from build123d import *

# Parameters (mm, degrees)
SKETCH1_W           = 30
SKETCH1_H           = 15
BOSS_EXTRUDE1_DEPTH = 15
SKETCH2_W           = 28
SKETCH2_H           = 13
CUT_EXTRUDE1_DEPTH  = 14
SKETCH3_R           = 1.5
CUT_EXTRUDE2_DEPTH  = 31
SKETCH4_R           = 1.5
CUT_EXTRUDE3_DEPTH  = 1


with BuildPart() as part:
    # Sketch1 → Boss-Extrude1 (new body)
    with BuildSketch(Plane(origin=(0, 0, 0), x_dir=(1, 0, 0), z_dir=(0, 1, 0))):
        Rectangle(SKETCH1_W, SKETCH1_H)
    extrude(amount=BOSS_EXTRUDE1_DEPTH)

    # Sketch2 → Cut-Extrude1 (cut)
    with BuildSketch(Plane(origin=(0, 15, 0), x_dir=(1, 0, 0), z_dir=(0, 1, 0))):
        Rectangle(SKETCH2_W, SKETCH2_H)
    extrude(amount=-CUT_EXTRUDE1_DEPTH, mode=Mode.SUBTRACT)

    # Sketch3 → Cut-Extrude2 (cut, through all)
    with BuildSketch(Plane(origin=(15, 0, 0), x_dir=(0, 0, -1), z_dir=(1, 0, 0))):
        with Locations((0, 7.5)):
            Circle(SKETCH3_R)
    extrude(amount=-CUT_EXTRUDE2_DEPTH, mode=Mode.SUBTRACT)

    # Sketch4 → Cut-Extrude3 (cut)
    with BuildSketch(Plane(origin=(0, 0, -7.5), x_dir=(-1, 0, 0), z_dir=(0, 0, -1))):
        with Locations((-7.5, 6.601224847)):
            Circle(SKETCH4_R)
        with Locations((7.5, 6.601224847)):
            Circle(SKETCH4_R)
    extrude(amount=-CUT_EXTRUDE3_DEPTH, mode=Mode.SUBTRACT)


solid = part.part
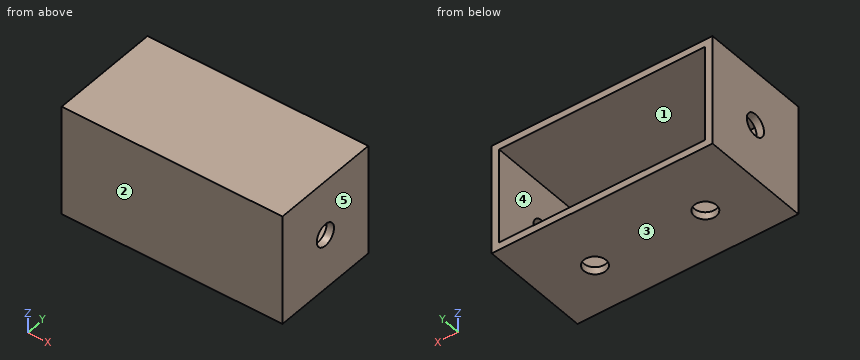
Could you check a few things on this model? Use its own coordinates, in mm. Face numbers are marked on the shaded views. A direction names the side the tool comes from. Coordinates: 2 decimals unless noted, no trailing zeros. Order: outer loops, then holes, each group sorted by start corner. A loop starts at its lowest first (then second) coordinate and runs counter-clockwise, first axis right, second up. Notation, with made-up numbers: (58, -10) -> (109, -10) arc R23 cw to (109, 16) -> close; hole circle Ø11 at (-6, 3). An arc over 180 degrees is marked (long way). One line per item, written item: value. Start each with the question number.
1) I'm going to push flat-ended pins straight in: pin 1 (3.5 mm diameter, centred on y = 7.5, z = 0, fed in from +X); pin 2 (4 mm diameter, centred on x = 5, z = 2, fed in from +Y). Where does each tip first touch, or does it pass through?
2) Imagine slicing it at C-C on y = 7.5. List the corners of the cut face in (x, z) for me.
3) We'd pull the mould along X, two halves only. Please class the marked faces 3, 4 and 5: +X half, -X half, draft (parallel to the pull), parting line (faces both ways), or undercut.
4) Imagine slicing it at D-D on y = 4.25. List the corners of the cut face in (x, z) for me, plus the area to 3 significant figures.
5) Imagine slicing it at B-B on x = -7.5. List the corners of the cut face in (y, z) for me, plus the area to 3 significant figures.
6) Which directions (+Z, -Z, +X, -X, +Y, -Y) give clear straight access to the entire face, cutting with the end or side of a thin tool? Please do the marked faces 1 and 2.
7) Imagine slicing it at A-A on z = 0. List the corners of the cut face in (x, y) for me, plus the area to 3 significant figures.
8) If I drill on L1, parallel to X at y = 1.25, z = 6.25; L2, parallel to Z at x = 7.5, y = 9.5; L3, parallel to Y at x = -7.5, z = -7, over which ranges is the centre line in solid material (lowest first)? Write a range as [from, to].
Answer list:
1. pin 1: stops at x = 15
1. pin 2: stops at y = 1
2. outline: (-15, -7.5) -> (-8.7, -7.5) -> (-8.7, -6.5) -> (-14, -6.5) -> (-14, -1.5) -> (-15, -1.5) -> close; (-15, 1.5) -> (-14, 1.5) -> (-14, 6.5) -> (14, 6.5) -> (14, 1.5) -> (15, 1.5) -> (15, 7.5) -> (-15, 7.5) -> close; (-6.3, -7.5) -> (6.3, -7.5) -> (6.3, -6.5) -> (-6.3, -6.5) -> close; (8.7, -7.5) -> (15, -7.5) -> (15, -1.5) -> (14, -1.5) -> (14, -6.5) -> (8.7, -6.5) -> close
3. face 3: draft
3. face 4: undercut
3. face 5: +X half
4. outline: (-15, -7.5) -> (15, -7.5) -> (15, 7.5) -> (-15, 7.5) -> close; hole (-14, -6.5) -> (14, -6.5) -> (14, 6.5) -> (-14, 6.5) -> close
4. area: 86.0 mm2
5. outline: (0, -7.5) -> (5.1, -7.5) -> (5.1, -6.5) -> (1, -6.5) -> (1, 6.5) -> (15, 6.5) -> (15, 7.5) -> (0, 7.5) -> close; (8.1, -7.5) -> (15, -7.5) -> (15, -6.5) -> (8.1, -6.5) -> close
5. area: 40.0 mm2
6. face 1: +Y
6. face 2: +Z, -Z, +X, -X, -Y
7. outline: (-15, 0) -> (15, 0) -> (15, 6) -> (14, 6) -> (14, 1) -> (-14, 1) -> (-14, 6) -> (-15, 6) -> close; (-15, 9) -> (-14, 9) -> (-14, 15) -> (-15, 15) -> close; (14, 9) -> (15, 9) -> (15, 15) -> (14, 15) -> close
7. area: 52.0 mm2
8. L1: x = [-15, -14], [14, 15]
8. L2: z = [-7.5, -6.5], [6.5, 7.5]
8. L3: y = [0, 5.1], [8.1, 15]
